Verification items for the finished model (mm, model axes). A direction names the side the tool comes from. Give positions to 0.01 mm unless a question says otherwise; leave off trailing zeros. Loops run counter-clockwise (first coordinate to the right, second up) from the corner with the lowest first, then second, coordinate; pieces in that order, holes last. Notation, with made-up numbers: (-38, 37) -> (0, 37) arc R13 ccw to (0, 42) -> close; hole circle Ø2 at (35.25, -10.75). An arc over 180 degrees is marked (long way). Use one line per item in the form item = value. Start each with the question number.
from build123d import *

# Parameters (mm, degrees)
SKETCH1_W                   = 196.85
SKETCH1_H                   = 82.55
BOSS_EXTRUDE1_DEPTH         = 95.25
SKETCH3_W                   = 146.05
SKETCH3_H                   = 76.2
CUT_EXTRUDE1_DEPTH          = 144.051280141
SKETCH4_W                   = 25.4
SKETCH4_H                   = 53.975
BOSS_EXTRUDE2_DEPTH         = 6.35
SKETCH5_W                   = 25.4
SKETCH5_H                   = 12.7
BOSS_EXTRUDE3_DEPTH         = 25.4
SKETCH6_W                   = 26.67
SKETCH6_H                   = 2.54
CUT_EXTRUDE2_DEPTH          = 229.622047548
F_1_4_0_25_DIAMETER_HOLE1_D = 6.35
SKETCH16_W                  = 196.85
SKETCH16_H                  = 6.35
CUT_EXTRUDE3_DEPTH          = 191.790819682
BOSS_EXTRUDE4_START         = -6.35
SKETCH11_W                  = 25.4
SKETCH11_H                  = 12.7
BOSS_EXTRUDE4_DEPTH         = 6.35
F_8_CLEARANCE_HOLE1_D       = 4.4958
F_8_CLEARANCE_HOLE1_DEPTH   = 12.7
SKETCH14_W                  = 146.05
SKETCH14_H                  = 41.275
BOSS_EXTRUDE5_DEPTH         = 6.35
M6X1_0_TAPPED_HOLE1_D       = 5
M6X1_0_TAPPED_HOLE1_DEPTH   = 14.986
M6X1_0_TAPPED_HOLE1_TIP     = 1.502151548


with BuildPart() as part:
    # Sketch1 → Boss-Extrude1 (new body)
    with BuildSketch(Plane(origin=(0, 0, 0), x_dir=(1, 0, 0), z_dir=(0, 1, 0))):
        Rectangle(SKETCH1_W, SKETCH1_H)
    extrude(amount=BOSS_EXTRUDE1_DEPTH)

    # Sketch3 → Cut-Extrude1 (cut, through all)
    with BuildSketch(Plane(origin=(0, 95.25, 0), x_dir=(1, 0, 0), z_dir=(0, 1, 0))):
        with Locations((0, -3.175)):
            Rectangle(SKETCH3_W, SKETCH3_H)
    extrude(amount=-CUT_EXTRUDE1_DEPTH, mode=Mode.SUBTRACT)

    # Sketch4 → Boss-Extrude2 (add)
    with BuildSketch(Plane(origin=(0, 0, -41.275), x_dir=(-1, 0, 0), z_dir=(0, 0, -1))):
        with Locations((-85.725, -26.9875)):
            Rectangle(SKETCH4_W, SKETCH4_H)
    boss_extrude2 = extrude(amount=-BOSS_EXTRUDE2_DEPTH)

    # Sketch5 → Boss-Extrude3 (add)
    with BuildSketch(Plane(origin=(0, 0, -41.275), x_dir=(-1, 0, 0), z_dir=(0, 0, -1))):
        with Locations((-85.725, -47.625)):
            Rectangle(SKETCH5_W, SKETCH5_H)
    boss_extrude3 = extrude(amount=BOSS_EXTRUDE3_DEPTH)

    # Sketch6 → Cut-Extrude2 (cut, through all)
    with BuildSketch(Plane(origin=(98.425, 0, 0), x_dir=(0, 0, -1), z_dir=(1, 0, 0))):
        with Locations((50.8, -52.705)):
            Rectangle(SKETCH6_W, SKETCH6_H)
    cut_extrude2 = extrude(amount=-CUT_EXTRUDE2_DEPTH, mode=Mode.SUBTRACT)

    # 1/4 (0.25) Diameter Hole1 (through all)
    with Locations(Plane(origin=(0, -41.275, 0), x_dir=(1, 0, 0), z_dir=(0, 1, 0))):
        with Locations((85.725, 53.975)):
            f_1_4_0_25_diameter_hole1 = Hole(F_1_4_0_25_DIAMETER_HOLE1_D / 2)

    # Sketch16 → Cut-Extrude3 (cut, through all)
    with BuildSketch(Plane(origin=(0, 95.25, 0), x_dir=(1, 0, 0), z_dir=(0, 1, 0))):
        with Locations((0, -38.1)):
            Rectangle(SKETCH16_W, SKETCH16_H)
    extrude(amount=-CUT_EXTRUDE3_DEPTH, mode=Mode.SUBTRACT)

    # Sketch11 → Boss-Extrude4 (add)
    with BuildSketch(Plane.XY.offset(41.275).offset(BOSS_EXTRUDE4_START)):
        with Locations((85.725, 101.6)):
            Rectangle(SKETCH11_W, SKETCH11_H)
        with Locations((85.725, -6.35)):
            Rectangle(SKETCH11_W, SKETCH11_H)
    boss_extrude4 = extrude(amount=-BOSS_EXTRUDE4_DEPTH)

    # #8 Clearance Hole1
    with Locations(Plane.XY.offset(41.275)):
        with Locations((85.725, 101.6), (85.725, -6.35)):
            f_8_clearance_hole1 = Hole(F_8_CLEARANCE_HOLE1_D / 2, depth=F_8_CLEARANCE_HOLE1_DEPTH)

    # Mirror1: Boss-Extrude2, Boss-Extrude3, Cut-Extrude2, 1/4 (0.25) Diameter Hole1, Boss-Extrude4, #8 Clearance Hole1 across plane
    add(boss_extrude2.mirror(Plane(origin=(0, 0, 0), x_dir=(0, 0, 1), z_dir=(1, 0, 0))))
    add(boss_extrude3.mirror(Plane(origin=(0, 0, 0), x_dir=(0, 0, 1), z_dir=(1, 0, 0))))
    add(cut_extrude2.mirror(Plane(origin=(0, 0, 0), x_dir=(0, 0, 1), z_dir=(1, 0, 0))), mode=Mode.SUBTRACT)
    add(f_1_4_0_25_diameter_hole1.mirror(Plane(origin=(0, 0, 0), x_dir=(0, 0, 1), z_dir=(1, 0, 0))), mode=Mode.SUBTRACT)
    add(boss_extrude4.mirror(Plane(origin=(0, 0, 0), x_dir=(0, 0, 1), z_dir=(1, 0, 0))))
    add(f_8_clearance_hole1.mirror(Plane(origin=(0, 0, 0), x_dir=(0, 0, 1), z_dir=(1, 0, 0))), mode=Mode.SUBTRACT)

    # Sketch14 → Boss-Extrude5 (add)
    with BuildSketch(Plane(origin=(0, 0, -41.275), x_dir=(-1, 0, 0), z_dir=(0, 0, -1))):
        with Locations((0, -20.6375)):
            Rectangle(SKETCH14_W, SKETCH14_H)
    extrude(amount=-BOSS_EXTRUDE5_DEPTH)

    # M6x1.0 Tapped Hole1
    with Locations(Plane(origin=(0, 0, -41.275), x_dir=(-1, 0, 0), z_dir=(0, 0, -1))):
        with Locations((-23, 79.416895565), (66, 79.416895565), (0, -8.333218687)):
            Hole(M6X1_0_TAPPED_HOLE1_D / 2, depth=M6X1_0_TAPPED_HOLE1_DEPTH)
            with Locations((0, 0, -(M6X1_0_TAPPED_HOLE1_DEPTH + M6X1_0_TAPPED_HOLE1_TIP / 2))):  # 118° drill point
                Cone(0, M6X1_0_TAPPED_HOLE1_D / 2, M6X1_0_TAPPED_HOLE1_TIP, mode=Mode.SUBTRACT)


solid = part.part
Item 1: Tool access check on faces 4 (the cylindrical face through (-87.97, 101.7, 31.71)), 5 (the flat face through (98.425, 26, -4)), 6 (the flat face through (-85.9, -51.435, -50.6)), 7 (the flat face through (-73.025, 47, 0)), 8 (the flat face through (89, -41.275, -51)). Record the directions out of +Z, -Z, +X, -X, +Y, -Y that give a thin tool (end or side, any length) a straight path to the whole face; none if there is none.
Item 2: Sectioned sample at B-B, the plane x = -66. Enter the section's corners in (y, z) (3 decimals).
Item 3: Gauge pin test, flat ends, axial feed: pin 1 Ø4 at (x, z) = (71.5, -24.5) entering from +Y; pin 2 Ø6 at (x, y) = (-13, 81) entering from +Z (3 decimals); pin 3 Ø6.5 at (x, y) = (-87, -5) entering from -Z (3 decimals); pin 4 Ø2.5 at (x, y) = (-85.725, 101.6) entering from -Z. Record the tip position at first contact, or that the pin passes through.
Item 4: Sectioned sample at D-D, the plane x = 76. Enter the section's corners in (y, z) (3 decimals).
Item 5: Material ranges on line 1 (X direction, y = 3.5, z = 27) (3 decimals); line 2 (X direction, y = 101, z = 33) (3 decimals); line 3 (Y direction, x = -66, z = -38.5) (3 decimals), recorded low to high.
Item 6: Sectioned sample at C-C, the plane y = 53. Enter the section's corners in (x, z) (3 decimals), and give its area (3 significant figures).
Item 7: Sectioned sample at A-A, the plane z = -46.5. Enter the section's corners in (x, y) (3 decimals).
Item 8: Draft check along Y on faces 1 (the flat face through (-86, 0, -4)), 2 (the cylindrical face through (87.509, 100.232, 31.706)), 3 (the cylindrical face through (-86.413, -46.426, -50.876)). Enter one of: +Y half, -Y half, draft (parallel to the pull), parting line (faces both ways), or undercut.
Outcome:
q1.face_4 = +Z, -Z
q1.face_5 = +Z, -Z, +X, +Y, -Y
q1.face_6 = +X, -X, -Y
q1.face_7 = +Z, +Y, -Y
q1.face_8 = -Z, +X, -X, +Y
q2.outline = (-41.275, -41.275) -> (76.917, -41.275) -> (76.917, -34.925) -> (-41.275, -34.925) -> close; (81.917, -41.275) -> (95.25, -41.275) -> (95.25, -34.925) -> (81.917, -34.925) -> close
q3.pin_1 = 95.25
q3.pin_2 = -34.925
q3.pin_3 = -41.275
q3.pin_4 = through
q4.outline = (-53.975, -66.675) -> (-41.275, -66.675) -> (-41.275, -41.275) -> (95.25, -41.275) -> (95.25, 28.575) -> (107.95, 28.575) -> (107.95, 34.925) -> (-12.7, 34.925) -> (-12.7, 28.575) -> (0, 28.575) -> (0, -34.925) -> (-53.975, -34.925) -> (-53.975, -37.465) -> (-51.435, -37.465) -> (-51.435, -64.135) -> (-53.975, -64.135) -> close
q5.line_1 = -98.425 to -73.025, 73.025 to 98.425
q5.line_2 = -98.425 to -87.891, -83.559 to -73.025, 73.025 to 83.559, 87.891 to 98.425
q5.line_3 = -41.275 to 76.917, 81.917 to 95.25
q6.outline = (-98.425, -41.275) -> (98.425, -41.275) -> (98.425, 34.925) -> (73.025, 34.925) -> (73.025, -34.925) -> (-73.025, -34.925) -> (-73.025, 34.925) -> (-98.425, 34.925) -> close
q6.area = 4,800 mm^2
q7.outline = (-98.425, -51.435) -> (-73.025, -51.435) -> (-73.025, -41.275) -> (-98.425, -41.275) -> close; (73.025, -51.435) -> (98.425, -51.435) -> (98.425, -41.275) -> (73.025, -41.275) -> close
q8.face_1 = -Y half
q8.face_2 = undercut
q8.face_3 = draft
